```python
from build123d import *

# Parameters (mm, degrees)
SKETCH_W     = 270.2
SKETCH_H     = 61
PAD_DEPTH    = 1.6
SKETCH001_W  = 1.6
SKETCH001_H  = 61
PAD001_DEPTH = 15
CHAMFER_SIZE = 1.5
FILLET_R     = 1.5
FILLET001_R  = 1.5
FILLET002_R  = 1


with BuildPart() as part:
    # Sketch → Pad (new body)
    with BuildSketch(Plane.XY):
        Rectangle(SKETCH_W, SKETCH_H)
    extrude(amount=PAD_DEPTH)

    # Sketch001 → Pad001 (join)
    with BuildSketch(Plane.XY):
        with Locations((-134.3, 0)):
            Rectangle(SKETCH001_W, SKETCH001_H)
        with Locations((134.3, 0)):
            Rectangle(SKETCH001_W, SKETCH001_H)
    extrude(amount=PAD001_DEPTH)

    # Chamfer
    chamfer_edges = [part.edges().sort_by_distance(p)[0] for p in [
        (-135.1, 30.5, 7.5),
        (135.1, 30.5, 7.5),
        (135.1, -30.5, 7.5),
        (-135.1, -30.5, 7.5),
    ]]
    chamfer(chamfer_edges, length=CHAMFER_SIZE)

    # Fillet
    fillet_edges = [part.edges().sort_by_distance(p)[0] for p in [
        (0, -30.5, 0),
        (0, 30.5, 0),
    ]]
    fillet(fillet_edges, radius=FILLET_R)

    # Fillet001
    fillet001_edges = [part.edges().sort_by_distance(p)[0] for p in [
        (-135.1, 0, 15),
        (135.1, 0, 15),
    ]]
    fillet(fillet001_edges, radius=FILLET001_R)

    # Fillet002
    fillet002_edges = [part.edges().sort_by_distance(p)[0] for p in [
        (-135.1, 0, 0),
        (135.1, 0, 0),
    ]]
    fillet(fillet002_edges, radius=FILLET002_R)


solid = part.part
```
The listing builds one solid part. Answer for the finished solid, in the listing's coordinates (mm). Coordinates: 2 decimals unless noted, no trailing zeros. Order: outer loops, then holes, each group sorted by start corner. A loop starts at its lowest first (then second) coordinate and runs counter-clockwise, first axis right, second up. Notation, with made-up numbers: M -17,-7 L 18,-7 A21 ccw 18,-1 Z; hole C 73,86 d5. An arc over 180 degrees is marked long. Answer as a JSON object with one key per item and string values. Group by question number.
1. Section C-C on x = 104 is taken. Write down the section's boundary in (y, z).
2. Section B-B on y = -19 is taken. Write down the section's boundary in (x, z), then the cut area to 3 significant figures.
3. Straight lines are drawn through the part: line 1 (X direction, y = -15, z = 13.75); line 2 (Z direction, x = 120, y = -8.5); line 3 (Y direction, x = -85, z = 0.75). For each, find the intervals that lie inside material, in ascending order.
4. Section A-A on z = 6.25 is taken. Write down the section's boundary in (x, y), then the cut area to 3 significant figures.
5. Determine the mould class of faces 1 (the flat face through (-2, 0, 0)), 2 (the flat face through (-2, 0, 1.6)), 3 (the flat face through (-135.1, 0, 7)), 4 (the flat face through (135.1, 0, 7)) for opening direction X: released by +X, released by -X, zero draft, split by the parting line, or undercut.
Values follow:
{
 "1": {"outline": "M -30.5,1.5 A1.5 ccw -29,0 L 29,0 A1.5 ccw 30.5,1.5 L 30.5,1.6 L -30.5,1.6 Z"},
 "2": {"outline": "M -135.1,1 A1 ccw -134.1,0 L 134.1,0 A1 ccw 135.1,1 L 135.1,13.5 A1.5 ccw 133.6,15 L 133.5,15 L 133.5,1.6 L -133.5,1.6 L -133.5,15 L -133.6,15 A1.5 ccw -135.1,13.5 Z", "area": "474 mm2"},
 "3": {"line 1": "-135.08 to -133.5, 133.5 to 135.08", "line 2": "0 to 1.6", "line 3": "-30.3 to 30.3"},
 "4": {"outline": "M -135.1,-29 L -133.6,-30.5 L -133.5,-30.5 L -133.5,30.5 L -133.6,30.5 L -135.1,29 Z; M 133.5,-30.5 L 133.6,-30.5 L 135.1,-29 L 135.1,29 L 133.6,30.5 L 133.5,30.5 Z", "area": "191 mm2"},
 "5": {"face 1": "zero draft", "face 2": "undercut", "face 3": "released by -X", "face 4": "released by +X"}
}
